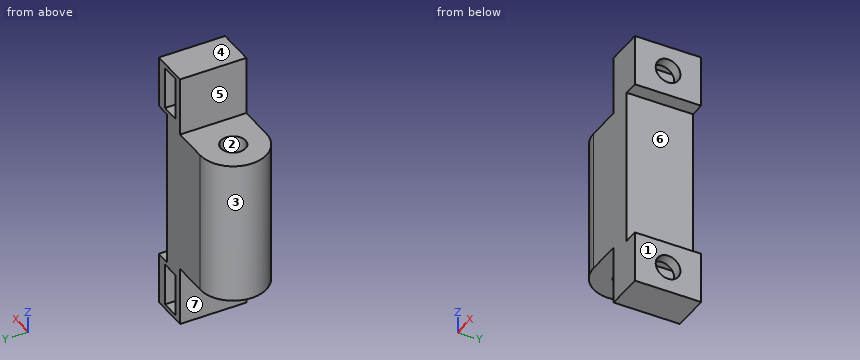
Autodesk Inventor part; units mm, degrees
ref_plane "YZ Plane" through (0, 0, 0) normal (1, 0, 0) x (0, 1, 0)
ref_plane "XZ Plane" through (0, 0, 0) normal (0, 1, 0) x (-1, 0, 0)
ref_plane "XY Plane" through (0, 0, 0) normal (0, 0, 1) x (1, 0, 0)
sketch "Эскиз1" plane through (0, 0, 0) normal (0, 0, 1) x (1, 0, 0)
  line L0 (0, 0) -> (8, 0)
  line L1 (8, 0) -> (8, 9)
  line L2 (8, 9) -> (0, 9)
  line L3 (0, 9) -> (0, 0)
  circle A0 centre (0, 4.5) radius 4.5
  dimension "d0" = 8
  dimension "d1" = 9
extrude "Выдавливание1" add sketch "Эскиз1" along normal blind 35.5
sketch "Эскиз2" plane through (8, 0, 0) normal (1, 0, 0) x (0, 0, -1)
  line L0 (-35.5, 0) -> (-35.5, 9)
  line L1 (0, 0) -> (-35.5, 0)
  line L2 (-35.5, 9) -> (-28.5, 9)
  line L3 (-28.5, 9) -> (-28.5, 0)
  line L4 (-28.5, 0) -> (-35.5, 0)
  line L5 (-35.5, 0) -> (-35.5, 9)
  line L6 (0, 0) -> (0, 9)
  line L7 (0, 9) -> (-7, 9)
  line L8 (-7, 9) -> (-7, 0)
  line L9 (-7, 0) -> (0, 0)
  line L10 (0, 0) -> (0, 9)
  dimension "d4" = 7
  dimension "d5" = 7
extrude "Выдавливание2" add sketch "Эскиз2" along normal blind 2
sketch "Эскиз3" plane through (10, 0, 0) normal (1, 0, 0) x (0, 0, -1)
  line L0 (-35.5, 9) -> (-35.5, 0)
  line L1 (-35.5, 4.5) -> (-28.5, 4.5)
  line L2 (-28.5, 0) -> (-28.5, 9)
  line L3 (-7, 9) -> (-7, 0)
  line L4 (-7, 4.5) -> (0, 4.5)
  line L5 (0, 9) -> (0, 0)
  point P0 (-32, 4.5)
  point P1 (-3.5, 4.5)
hole "Отверстие1" at (10, 4.5, 32) at (10, 4.5, 3.5) direction (-1, 0, 0) diameter 3.35 depth 4
sketch "Эскиз4" plane through (10, 0, 0) normal (1, 0, 0) x (0, 0, -1)
  circle A0 centre (-32, 4.5) radius 1.675
  line L0 (-34.9, 6.1743) -> (-32, 7.8486)
  line L1 (-32, 7.8486) -> (-29.1, 6.1743)
  line L2 (-29.1, 6.1743) -> (-29.1, 2.8257)
  line L3 (-29.1, 2.8257) -> (-32, 1.1514)
  line L4 (-32, 1.1514) -> (-34.9, 2.8257)
  line L5 (-34.9, 2.8257) -> (-34.9, 6.1743)
  circle A1 centre (-3.5, 4.5) radius 1.675
  line L6 (-6.4, 6.1743) -> (-3.5, 7.8486)
  line L7 (-3.5, 7.8486) -> (-0.6, 6.1743)
  line L8 (-0.6, 6.1743) -> (-0.6, 2.8257)
  line L9 (-0.6, 2.8257) -> (-3.5, 1.1514)
  line L10 (-3.5, 1.1514) -> (-6.4, 2.8257)
  line L11 (-6.4, 2.8257) -> (-6.4, 6.1743)
  line L12 (0, 9) -> (-35.5, 9)
  line L13 (-6.4, 6.1743) -> (-0.6, 6.1743)
  line L14 (-0.6, 6.1743) -> (-0.6, 9)
  line L15 (-0.6, 9) -> (-6.4, 9)
  line L16 (-6.4, 9) -> (-6.4, 6.1743)
  line L17 (-29.1, 6.1743) -> (-34.9, 6.1743)
  line L18 (-34.9, 6.1743) -> (-34.9, 9)
  line L19 (-34.9, 9) -> (-29.1, 9)
  line L20 (-29.1, 9) -> (-29.1, 6.1743)
  point P0 (0, 0)
  dimension "d15" = 5.8
  dimension "d16" = 5.8
extrude "Выдавливание3" cut sketch "Эскиз4" along normal blind 2.5 from surface at -4
sketch "Эскиз5" plane through (0, 0, 35.5) normal (0, 0, 1) x (1, 0, 0)
  line L0 (0, 9) -> (10, 9)
  circle A0 centre (0, 4.5) radius 4.5
  arc A1 (0, 9) -> (0, 0) centre (0, 4.5) ccw
  line L1 (0, 9) -> (4.85, 9)
  line L2 (4.85, 9) -> (4.85, 0)
  line L3 (4.85, 0) -> (0, 0)
  line L4 (0, 0) -> (0, 9)
  point P0 (0, 0)
  dimension "d40" = 9
  dimension "d41" = 4.85
extrude "Выдавливание4" cut sketch "Эскиз5" against normal blind 8
sketch "Эскиз6" plane through (0, 0, 0) normal (0, 0, -1) x (-1, 0, 0)
  circle A0 centre (0, 4.5) radius 4.5
  line L0 (0, 9) -> (-10, 9)
  line L1 (0, 9) -> (-4.85, 9)
  line L2 (-4.85, 9) -> (-4.85, 0)
  line L3 (-4.85, 0) -> (0, 0)
  line L4 (0, 0) -> (0, 9)
  point P0 (0, 0)
  dimension "d42" = 9
  dimension "d43" = 4.85
extrude "Выдавливание5" cut sketch "Эскиз6" against normal blind 8
sketch "Эскиз7" plane through (0, 0, 8) normal (0, 0, -1) x (-1, 0, 0)
  arc A0 (0, 0) -> (0, 9) centre (0, 4.5) ccw
hole "Отверстие2" at (0, 4.5, 8) direction (0, 0, 1) diameter 3.35 end through all
equation "\"d16\" = d15"
properties part number "Крепление Open MV"
Part model, mm, in its own coordinate system. Face numbers are marked on the shaded views. A direction names the side the tool comes from. Give positions to 0.01 mm unless a question says otherwise; leave off trailing zeros. Order: outer loops, then holes, each group sorted by start corner. A loop starts at its lowest first (then second) coordinate and runs counter-clockwise, first axis right, second up. Notation, with made-up numbers: (-1.5, -27) - (34.5, -27) arc R27 ccw to (34.5, 6) - close; hole circle Ø4 at (8, -1.5). An arc over 180 degrees is marked (long way). One line per question, with ' | ' between items.
1. Band-saw the part on D-D on x = 4. List the corners of the cut face in (y, z).
Filled in:
outline: (0, 8) - (9, 8) - (9, 27.5) - (0, 27.5) - close
2. Band-saw the part on C-C on z = 15.5. List the corners of the cut face in (x, y) (3 decimals), then the cut area to 3 significant figures.
Filled in:
outline: (0, 0) - (8, 0) - (8, 9) - (0, 9) arc R4.5 ccw to start; hole circle Ø3.35 at (0, 4.5) | area: 95.0 mm²
3. Which spindle directions (+Z, -Z, +X, -X, +Y, -Y) get a long thin tool onto all of the face, cutting with end or side? Do the marked faces 4, 5, 6 and 7. Say none if no direction does.
Filled in:
face 4: +Z, +X, -X, +Y, -Y | face 5: +Z, -X, +Y, -Y | face 6: +X, +Y, -Y | face 7: -Z, -X, +Y, -Y
4. Drill centre lines: probe 1 along Z at (x, y) = (6.25, 3); probe 2 along Z at (x, y) = (9.5, 4.5) (3 decimals); probe 3 along Y at (x, z) = (8.9, 32) (3 decimals). Where is each one in solid material? Low to high.
Filled in:
probe 1: 0 to 0.6, 6.4 to 29.1, 34.9 to 35.5 | probe 2: 0 to 1.825, 5.175 to 7, 28.5 to 30.325, 33.675 to 35.5 | probe 3: 0 to 2.825, 6.175 to 9
5. Drop a flat-ended pin along its axis: P1, Ø3, axis at y = 4, z = 32.5, coming from the -X side. Give the stop position or say it passes through.
Filled in:
P1: x = 4.85
6. Band-saw the part on B-B on z = 32.5. List the corners of the cut face in (x, y).
Filled in:
outline: (4.85, 0) - (10, 0) - (10, 2.9) - (8.5, 2.9) - (8.5, 1.44) - (6, 1.44) - (6, 9) - (4.85, 9) - close; (8.5, 6.1) - (10, 6.1) - (10, 9) - (8.5, 9) - close
7. Pull direction X, two halves, no side cores. Call the marked faces 1, 2 and 3: +X half, -X half, draft (parallel to the pull), parting line (faces both ways), or undercut.
Filled in:
face 1: +X half | face 2: undercut | face 3: -X half
